from build123d import *

# Parameters (mm, degrees)
EXTRUDE_1_DEPTH        = 19.95
HOLE_WIZARD_M3_1_D     = 2.5
HOLE_WIZARD_M3_1_DEPTH = 4.5
HOLE_WIZARD_M3_1_TIP   = 0.751075774


with BuildPart() as part:
    # 草图1 → 凸台-拉伸1 (new, symmetric)
    with BuildSketch(Plane(origin=(0, 0, 0), x_dir=(0, 0, -1), z_dir=(1, 0, 0))):
        Polygon((0, 0), (0, 8), (20, 8), (20, 0), (14.5, 0), (14.5, 4.5), (5.5, 4.5), (5.5, 0), align=None)
    extrude(amount=EXTRUDE_1_DEPTH, both=True)

    # M3 螺纹孔1
    with Locations(Plane(origin=(0, 8, 0), x_dir=(1, 0, 0), z_dir=(0, 1, 0))):
        with Locations((-8, 17.5), (8, 17.5), (8, 2.5), (-8, 2.5)):
            Hole(HOLE_WIZARD_M3_1_D / 2, depth=HOLE_WIZARD_M3_1_DEPTH)
            with Locations((0, 0, -(HOLE_WIZARD_M3_1_DEPTH + HOLE_WIZARD_M3_1_TIP / 2))):  # 118° drill point
                Cone(0, HOLE_WIZARD_M3_1_D / 2, HOLE_WIZARD_M3_1_TIP, mode=Mode.SUBTRACT)


solid = part.part
The listing builds one solid part. Answer for the finished solid, in the listing's coordinates (mm). A direction names the side the tool comes from. Round coordinates to 2 decimals unless told otherwise and drop trailing zeros. Write each loop counter-clockwise with the first axis right and the second up, starting at its lowest first coordinate (ties: lowest second). Pieces come first, ordered by that corner, then holes. Notation, with made-up numbers: M 2,25 L 49,25 A25 ccw 49,51 Z; hole C -18.75,88.25 d6. An arc over 180 degrees is marked long. Write each question's results on one line, items separated by ' | '. Start each with the question number.
Item 1: Find section B-B on y = 4. Write down the section's boundary in (x, z).
Item 2: Find section C-C on y = 6.5. Write down the section's boundary in (x, z), and give its area (3 significant figures).
Item 3: Find section D-D on x = 11. Write down the section's boundary in (y, z).
Item 4: Which of the six approach directions +Z, -Z, +X, -X, +Y, -Y give full straight-line access (tool end or side, diameter ignored) to faces 1 (the flat face through (0, 8, -10)), 2 (the flat face through (0, 2, -14.5)), 3 (the cylindrical face through (9.25, 5.72, -2.55))?
Item 5: Straight lines are drawn through the part: probe 1 along X at (y, z) = (5.65, -17.5); probe 2 along Z at (x, y) = (7, 0.5); probe 3 along X at (y, z) = (4.5, -16.75). For each, find the intervals that lie inside material, in ascending order.
Item 6: Given pin 1 Ø2 at (x, z) = (8, -2.5) entering from +Y, flat-ended and moving along its own axis, determine where the tip first touches the part or whether it passes through.
Item 7: Find section A-A on y = 1.5. Write down the section's boundary in (x, z), and give its area (3 significant figures).
Item 8: The mould has two halves that part along Z. Classify faces 4 (the flat face through (0, 4, 0)), 5 (the flat face through (0, 2, -5.5)), 6 (the flat face through (0, 0, -3)): +Z half, -Z half, draft (parallel to the pull), parting line (faces both ways), or undercut.
Answer block:
1) outline: M -19.95,-20 L 19.95,-20 L 19.95,-14.5 L -19.95,-14.5 Z; M -19.95,-5.5 L 19.95,-5.5 L 19.95,0 L -19.95,0 Z; hole C -8,-17.5 d2.5; hole C -8,-2.5 d2.5; hole C 8,-17.5 d2.5; hole C 8,-2.5 d2.5
2) outline: M -19.95,-20 L 19.95,-20 L 19.95,0 L -19.95,0 Z; hole C -8,-17.5 d2.5; hole C -8,-2.5 d2.5; hole C 8,-17.5 d2.5; hole C 8,-2.5 d2.5 | area: 778 mm²
3) outline: M 0,-20 L 8,-20 L 8,0 L 0,0 L 0,-5.5 L 4.5,-5.5 L 4.5,-14.5 L 0,-14.5 Z
4) face 1: +Z, -Z, +X, -X, +Y | face 2: +X, -X, -Y | face 3: +Y
5) probe 1: x = -19.95 to -9.25, -6.75 to 6.75, 9.25 to 19.95 | probe 2: z = -20 to -14.5, -5.5 to 0 | probe 3: x = -19.95 to -9, -7 to 7, 9 to 19.95
6) pin 1: stops at y = 3.35
7) outline: M -19.95,-20 L 19.95,-20 L 19.95,-14.5 L -19.95,-14.5 Z; M -19.95,-5.5 L 19.95,-5.5 L 19.95,0 L -19.95,0 Z | area: 439 mm²
8) face 4: +Z half | face 5: undercut | face 6: draft
